Geometry check sheet. Reference: drawing and pictorial views, mm from the part's lowest x, y, z. Coordinates: 2 decimals unless noted, no trailing zeros. Write each loop counter-clockwise with the first axis right and the second up, starting at its lowest first coordinate (ties: lowest second). Pieces come first, ordered by that corner, then holes. Notation, with made-up numbers: (10, -13) -> (27, -13) arc R20 ccw to (27, 5) -> close; hole circle Ø3 at (79.25, -13.5). An arc over 180 degrees is marked (long way). Use a Markdown table: item, result.
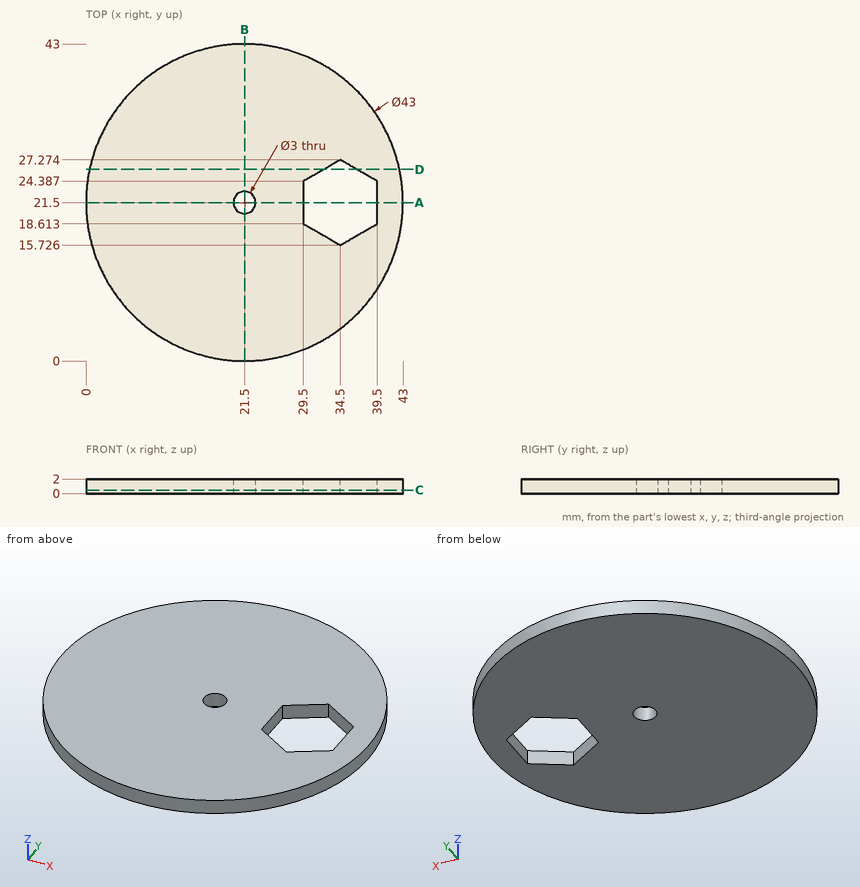
Item 1: Thickness scan on L1, parallel to Y at x = 21.5, z = 1.6; L2, parallel to X at y = 22, z = 0.5 (1 decimal); L3, parallel to X at y = 27, z = 0.25 (1 decimal). Record the ranges inside material, lowest first. Write a range as [from, to].
Answer block:
| item | result |
|---|---|
| L1 | y = [0, 20], [23, 43] |
| L2 | x = [0, 20.1], [22.9, 29.5], [39.5, 43] |
| L3 | x = [0.7, 34], [35, 42.3] |
Item 2: Depth check by flat-ended pin: P1, Ø1, axis at x = 33, z = 0.5, coming from the -Y side. Enter the tip coordinate at first touch or a pass-through.
Answer block:
| item | result |
|---|---|
| P1 | stops at y = 3.03 |
Item 3: Section check D-D on y = 26. Record the boundary of the cut face in (x, z) (1 decimal).
Answer block:
| item | result |
|---|---|
| outline | (0.5, 0) -> (32.3, 0) -> (32.3, 2) -> (0.5, 2) -> close; (36.7, 0) -> (42.5, 0) -> (42.5, 2) -> (36.7, 2) -> close |
Item 4: Section check B-B on x = 21.5. Record the boundary of the cut face in (y, z).
Answer block:
| item | result |
|---|---|
| outline | (0, 0) -> (20, 0) -> (20, 2) -> (0, 2) -> close; (23, 0) -> (43, 0) -> (43, 2) -> (23, 2) -> close |
Item 5: Section check A-A on y = 21.5. Record the boundary of the cut face in (x, z).
Answer block:
| item | result |
|---|---|
| outline | (0, 0) -> (20, 0) -> (20, 2) -> (0, 2) -> close; (23, 0) -> (29.5, 0) -> (29.5, 2) -> (23, 2) -> close; (39.5, 0) -> (43, 0) -> (43, 2) -> (39.5, 2) -> close |
Item 6: Section check C-C on z = 0.5. Record the boundary of the cut face in (x, y), then the cut area to 3 significant figures.
Answer block:
| item | result |
|---|---|
| outline | circle Ø43 at (21.5, 21.5); hole circle Ø3 at (21.5, 21.5); hole (29.5, 18.61) -> (34.5, 15.73) -> (39.5, 18.61) -> (39.5, 24.39) -> (34.5, 27.27) -> (29.5, 24.39) -> close |
| area | 1,360 mm^2 |
